from build123d import *

# Parameters (mm, degrees)
SKETCH1_W           = 35
SKETCH1_H           = 35
BOSS_EXTRUDE1_DEPTH = 36.3
SKETCH2_R           = 11
BOSS_EXTRUDE2_DEPTH = 2
BOSS_EXTRUDE4_DEPTH = 14.2


with BuildPart() as part:
    # Sketch1 → Boss-Extrude1 (new body)
    with BuildSketch(Plane(origin=(0, 0, 0), x_dir=(0, 0, -1), z_dir=(1, 0, 0))):
        with Locations((-17.5, -17.5)):
            Rectangle(SKETCH1_W, SKETCH1_H)
    extrude(amount=BOSS_EXTRUDE1_DEPTH)

    # Sketch2 → Boss-Extrude2 (add)
    with BuildSketch(Plane.ZY):
        with Locations((17.5, -17.5)):
            Circle(SKETCH2_R)
    extrude(amount=BOSS_EXTRUDE2_DEPTH)

    # Sketch3 → Boss-Extrude4 (add)
    with BuildSketch(Plane.ZY.offset(2)):
        with BuildLine():
            Line((17.5, -15.55), (19.064448785, -15.55))
            ThreePointArc((19.064448785, -15.55), (17.5, -20), (15.935551215, -15.55))
            Line((15.935551215, -15.55), (17.5, -15.55))
        make_face()
    extrude(amount=BOSS_EXTRUDE4_DEPTH)


solid = part.part
Work out the finished part from the listing and answer in its coordinate system (mm). A direction names the side the tool comes from. Give positions to 0.01 mm unless a question says otherwise; leave off trailing zeros. Loops run counter-clockwise (first coordinate to the right, second up) from the corner with the lowest first, then second, coordinate; pieces in that order, holes last. Notation, with made-up numbers: (-2.5, 65) - (18.5, 65) arc R23 cw to (18.5, 81) - close; hole circle Ø5 at (-25.75, -23). An arc over 180 degrees is marked (long way). Answer in a Markdown table with one row per item. Add a question column.
Q1. The part is cut by section A-A (y = -17.5). Determine the outline of the cut face in (x, z).
Q2. A tool of negligible diameter and unlimited length cuts with its end or side. For faces 1 (the flat face through (18, -35, 18)), 2 (the cylindrical face through (-0.986, -27.259, 22.576)), 3 (the flat face through (-9, -15.55, 17)), from which of +Z, -Z, +X, -X, +Y, -Y can it reach the whole face along a straight path? Write none if from no direction.
Q3. Each of these flat-tipped pins is pushed along its axis until it touches: P1, Ø3, axis at y = -21.5, z = 10.5, coming from the -X side; P2, Ø1.6, axis at x = -7, z = 18, coming from the +Y side. Where does it stop, or does it pass through?
Q4. The part is cut by section C-C (x = -3.5). Determine the outline of the cut face in (y, z).
Q5. The part is cut by section B-B (z = 17.5). Determine the outline of the cut face in (x, y), and give its area (3 significant figures).
Q6. Consider line 1 along X through (y, z) = (-13.5, 20.5); line 2 along X through (y, z) = (-10, 32.5); line 3 along Z through (x, y) = (-10, -16). Determine where each line is inside the solid, lowest interval first.
Q7. The part is cut by section D-D (z = 11). Determine the outline of the cut face in (x, y).
Solution:
| question | item | result |
|---|---|---|
| 1 | outline | (-16.2, 15) - (-2, 15) - (-2, 6.5) - (0, 6.5) - (0, 0) - (36.3, 0) - (36.3, 35) - (0, 35) - (0, 28.5) - (-2, 28.5) - (-2, 20) - (-16.2, 20) - close |
| 2 | face 1 | +Z, -Z, +X, -X, -Y |
| 2 | face 2 | -X |
| 2 | face 3 | +Z, -Z, -X, +Y |
| 3 | P1 | stops at x = -2 |
| 3 | P2 | stops at y = -15.55 |
| 4 | outline | (-15.55, 15.94) - (-15.55, 19.06) arc R2.5 ccw (long way) to start |
| 5 | outline | (-16.2, -20) - (-2, -20) - (-2, -28.5) - (0, -28.5) - (0, -35) - (36.3, -35) - (36.3, 0) - (0, 0) - (0, -6.5) - (-2, -6.5) - (-2, -15.55) - (-16.2, -15.55) - close |
| 5 | area | 1,380 mm² |
| 6 | line 1 | x = -2 to 36.3 |
| 6 | line 2 | x = 0 to 36.3 |
| 6 | line 3 | z = 15.5 to 19.5 |
| 7 | outline | (-2, -26.37) - (0, -26.37) - (0, -35) - (36.3, -35) - (36.3, 0) - (0, 0) - (0, -8.63) - (-2, -8.63) - close |
